Could you check a few things on this model? Use its own coordinates, in mm. A direction names the side the tool comes from. Give positions to 0.01 mm unless a question says otherwise; leave off trailing zeros. Order: outer loops, then holes, each group sorted by start corner. A loop starts at its lowest first (then second) coordinate and runs counter-clockwise, first axis right, second up. Notation, with made-up numbers: M 85,23 L 139,23 A22 ccw 139,45 Z; hole C -36.75,-15.75 d11. An arc over 180 degrees is marked long. Use a Markdown table: item, result. Add a question column.
Item 1: For faces 5 (the face through (-1.168, -0.644, 24.85)), 6 (the face through (4.736, -0.76, 12.332)), 7 (the face through (2, 0, 13)), which set-ups out of +Z, -Z, +X, -X, +Y, -Y let a thin tool reach every point of the face, with its end or its side?
Item 2: If I drill on L1, parallel to Z at x = 4.5, y = -0.4; L2, parallel to Z at x = 5.25, y = -0.75; L3, parallel to X at y = -1.4, z = 16, over which ranges is the centre line in solid material (lowest first)? Write a range as from..to.
Item 3: Suppose I cut it at A-A on z = 14.5. Write out the boundary of the cut face in (x, y), plus the area to 3 significant figures.
Item 4: If we mould it in two halves opening along Z, with no side actions, what happens to faces 1 (the face through (5.4, -0.2, 25)), 2 (the face through (2, -1, -1)), 3 (the face through (5.792, -0.8, 25.4)), 4 (the face through (2, -1, 26))? For each: released by +Z, released by -Z, zero draft, split by the parting line, or undercut.
from build123d import *

# Parameters (mm, degrees)
BOSS_EXTRUDE1_DEPTH = 25
SKETCH2_W           = 7.93444402
SKETCH2_H           = 1.5
BOSS_EXTRUDE2_DEPTH = 1
SKETCH3_W           = 7.93444402
SKETCH3_H           = 1.5
BOSS_EXTRUDE3_DEPTH = 1
FILLET1_R           = 0.5


with BuildPart() as part:
    # Sketch1 → Boss-Extrude1 (new body)
    with BuildSketch(Plane.XY):
        Polygon((0, 0), (-2.14222201, -1.5), (5.79222201, -1.5), (3.65, 0), align=None)
    extrude(amount=BOSS_EXTRUDE1_DEPTH)

    # Sketch2 → Boss-Extrude2 (add)
    with BuildSketch(Plane.XY.offset(25)):
        with Locations((1.825, -0.75)):
            Rectangle(SKETCH2_W, SKETCH2_H)
    extrude(amount=BOSS_EXTRUDE2_DEPTH)

    # Sketch3 → Boss-Extrude3 (add)
    with BuildSketch(Plane(origin=(0, 0, 0), x_dir=(-1, 0, 0), z_dir=(0, 0, -1))):
        with Locations((-1.825, -0.75)):
            Rectangle(SKETCH3_W, SKETCH3_H)
    extrude(amount=BOSS_EXTRUDE3_DEPTH)

    # Fillet1
    fillet1_edges = [part.edges().sort_by_distance(p)[0] for p in [
        (4.721111005, -0.75, 25),
        (4.721111005, -0.75, 0),
        (-1.071111005, -0.75, 0),
        (-1.071111005, -0.75, 25),
    ]]
    fillet(fillet1_edges, radius=FILLET1_R)


solid = part.part
Findings below:
| question | item | result |
|---|---|---|
| 1 | face 5 | -X, +Y |
| 1 | face 6 | +X, +Y |
| 1 | face 7 | +Z, -Z, +X, -X, +Y |
| 2 | L1 | z = -1..0.13, 24.87..26 |
| 2 | L2 | z = -1..0.04, 24.96..26 |
| 2 | L3 | x = -2..5.65 |
| 3 | outline | M -2.14,-1.5 L 5.79,-1.5 L 3.65,0 L 0,0 Z |
| 3 | area | 8.69 mm^2 |
| 4 | face 1 | undercut |
| 4 | face 2 | released by -Z |
| 4 | face 3 | zero draft |
| 4 | face 4 | released by +Z |
